Check sheet for the drawn part. Datum: minimum x, y, z corner. Units: mm. A direction names the side the tool comes from. Coordinates: 2 decimals unless noted, no trailing zeros. Write each loop counter-clockwise with the first axis right and the second up, starting at its lowest first coordinate (ties: lowest second). Pieces come first, ordered by that corner, then holes. Notation, with made-up numbers: (-20, 39.25) -> (39, 39.25) arc R25 cw to (39, 64.25) -> close; hole circle Ø2 at (45, -3.75). An arc over 180 degrees is marked (long way). Answer in a Markdown table with one row per item. Add a question column.
1. Set-up check for the marked faces 1 and 2: record each of +Z, -Z, +X, -X, +Y, -Y from which the full face is reachable in a straight line by a thin tool's end or side.
2. Cross-section at B-B on x = 16. Record the cut outline in (y, z), and give its area (3 significant figures).
3. Cross-section at A-A on z = 1.95. Record the cut outline in (x, y).
4. Scan lines: L1, parallel to X at y = 17.25, z = 1.05; L2, parallel to Y at x = 10.25, z = 0.5. Record each from-to range of solid material in increasing order. Write a range as from..to.
5. Depth check by flat-ended pin: P1, Ø1.8, axis at y = 15.5, z = 3.5, coming from the +X side; P2, Ø3, axis at x = 16, z = 2.5, coming from the +Y side; P3, Ø1.5, axis at y = 9, z = 1.5, coming from the +X side; P4, Ø1.5, axis at y = 15, z = 0.5, coming from the -X side. Enter the tip coordinate at first touch or a pass-through.
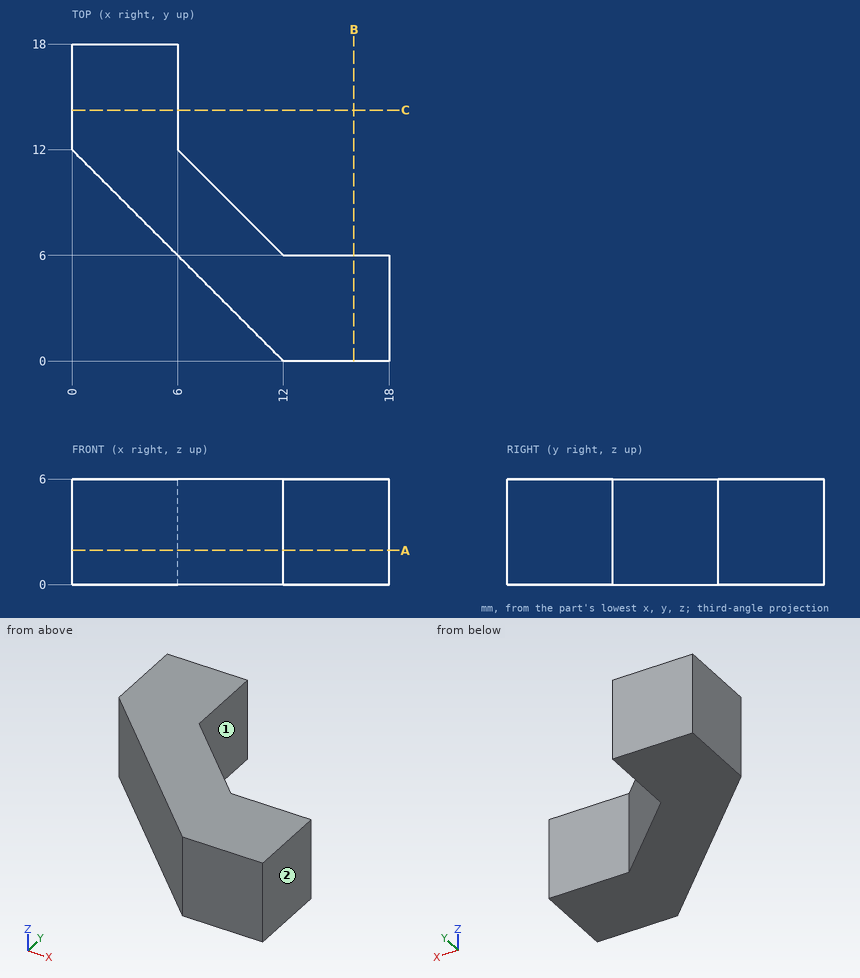
Results found:
| question | item | result |
|---|---|---|
| 1 | face 1 | +Z, -Z, +X, +Y |
| 1 | face 2 | +Z, -Z, +X, +Y, -Y |
| 2 | outline | (0, 0) -> (6, 0) -> (6, 6) -> (0, 6) -> close |
| 2 | area | 36.0 mm^2 |
| 3 | outline | (0, 12) -> (12, 0) -> (18, 0) -> (18, 6) -> (12, 6) -> (6, 12) -> (6, 18) -> (0, 18) -> close |
| 4 | L1 | x = 0..6 |
| 4 | L2 | y = 1.75..7.75 |
| 5 | P1 | stops at x = 6 |
| 5 | P2 | stops at y = 6 |
| 5 | P3 | stops at x = 9.75 |
| 5 | P4 | stops at x = 0 |
